from build123d import *

# Parameters (mm, degrees)
SKETCH_1_R          = 6
EXTRUDE_1_DEPTH     = 6
CUT_EXTRUDE_1_DEPTH = 5
CHAMFER_1_SIZE      = 1


with BuildPart() as part:
    # 草图1 → 凸台-拉伸1 (new body)
    with BuildSketch(Plane(origin=(0, 0, 0), x_dir=(1, 0, 0), z_dir=(0, 1, 0))):
        with Locations(Location((0, 0, 0), (0, 0, 270))):
            Circle(SKETCH_1_R)
    extrude(amount=EXTRUDE_1_DEPTH)

    # 草图2 → 切除-拉伸1 (cut)
    with BuildSketch(Plane(origin=(0, 6, 0), x_dir=(1, 0, 0), z_dir=(0, 1, 0))):
        Polygon((1.261535508, 3.20868814), (-2.148037688, 2.696865868), (-3.409573196, -0.511822272), (-1.261535508, -3.20868814), (2.148037688, -2.696865868), (3.409573196, 0.511822272), align=None)
    extrude(amount=-CUT_EXTRUDE_1_DEPTH, mode=Mode.SUBTRACT)

    # 倒角1
    chamfer_1_edges = [part.edges().sort_by_distance(p)[0] for p in [
        (0, 6, -6),
    ]]
    chamfer(chamfer_1_edges, length=CHAMFER_1_SIZE)


solid = part.part
CAD build for the part. Positions are in the model's coordinates, mm. A direction names the side the tool comes from. Coordinates: 2 decimals unless noted, no trailing zeros. Write each loop counter-clockwise with the first axis right and the second up, starting at its lowest first coordinate (ties: lowest second). Pieces come first, ordered by that corner, then holes. Notation, with made-up numbers: M 56,34 L 103,34 A25 cw 103,65 Z; hole C -7.5,1.25 d1. An arc over 180 degrees is marked long. Answer as a JSON object with one key per item and string values. Group by question number.
1) Mould opens along X. For faces 3 (the face through (0.1, 6, 3.3)), 4 (the face through (-2.77, 3.54, -1.11)), 5 (the face through (1.802, 2.465, 5.723)) say: +X half, -X half, draft (parallel to the pull), parting line (faces both ways), or undercut.
2) Saw through at B-B (z = 0). Write the cut outline in (x, y).
3) Tool access for faces 1 (the face through (-0.419, 3.535, -2.956)), 2 (the face through (0, 0, 0)): list every direction of +Z, -Z, +X, -X, +Y, -Y with a clear straight run to the whole face (end or side of a thin tool).
4) Saw through at D-D (x = 0). Write the cut outline in (y, z), plus the area to 3 significant figures.
5) Pin check, flat tip, straight feed: pin 1 Ø1.5 at (y, z) = (2, -4.5) entering from +X. Stop position of the tip, or through.
6) Wall check: line 1 (X direction, y = 1.2, z = 1.75); line 2 (Y direction, x = 0.5, z = -0.5); line 3 (Z direction, x = -0.25, y = 4.4). Give the ranges that are in metal, low to high. Write a range as from..to.
7) Saw through at A-A (y = 4.3). Write the cut outline in (x, z).
8) Saw through at C-C (y = 0.7). Write the cut outline in (x, z).
Values follow:
{
 "1": {"face 3": "draft", "face 4": "undercut", "face 5": "parting line"},
 "2": {"outline": "M -6,0 L 6,0 L 6,5 L 5,6 L 3.21,6 L 3.21,1 L -3.21,1 L -3.21,6 L -5,6 L -6,5 Z"},
 "3": {"face 1": "+Y", "face 2": "+Z, -Z, +X, -X, -Y"},
 "4": {"outline": "M 0,-6 L 5,-6 L 6,-5 L 6,-3.02 L 1,-3.02 L 1,3.02 L 6,3.02 L 6,5 L 5,6 L 0,6 Z", "area": "40.8 mm2"},
 "5": {"pin 1": "stops at x = 4.68"},
 "6": {"line 1": "x = -5.74..-2.42, 2.52..5.74", "line 2": "y = 0..1", "line 3": "z = -5.99..-2.98, 3.06..5.99"},
 "7": {"outline": "C 0,0 d12; hole M -3.41,0.51 L -2.15,-2.7 L 1.26,-3.21 L 3.41,-0.51 L 2.15,2.7 L -1.26,3.21 Z"},
 "8": {"outline": "C 0,0 d12"}
}
